Design review of the part shown in the three views and the two pictorial views. Dimensions are in mm from the part's minimum x, y and z. A direction names the side the tool comes from. Give positions to 0.01 mm unless a question says otherwise; leave off trailing zeros. Order: outer loops, then holes, each group sorted by start corner. A loop starts at its lowest first (then second) coordinate and runs counter-clockwise, first axis right, second up.
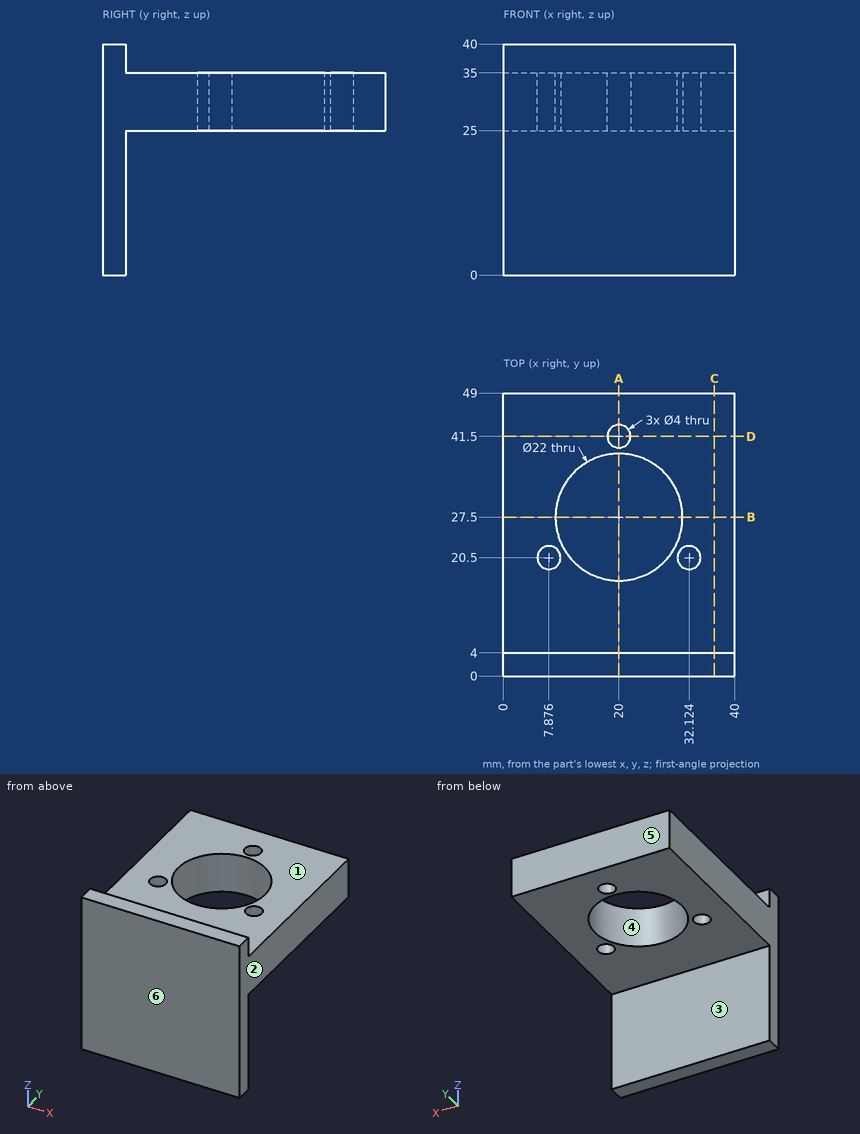
Item 1: For line 1 (Y direction, x = 20, z = 31.5); line 2 (X direction, y = 20, z = 29) (1 decimal); line 3 (X direction, y = 27, z = 30), list the stretches that pass through material, from the lowest coordinate up.
Values found:
line 1: y = 0 to 16.5, 38.5 to 39.5, 43.5 to 49
line 2: x = 0 to 5.9, 9.8 to 12, 28 to 30.2, 34.1 to 40
line 3: x = 0 to 9.01, 30.99 to 40
Item 2: Take a section at A-A (x = 20). Give the boundary of the cut face in (y, z), and give its area (3 significant figures).
Values found:
outline: (0, 0) - (4, 0) - (4, 25) - (16.5, 25) - (16.5, 35) - (4, 35) - (4, 40) - (0, 40) - close; (38.5, 25) - (39.5, 25) - (39.5, 35) - (38.5, 35) - close; (43.5, 25) - (49, 25) - (49, 35) - (43.5, 35) - close
area: 350 mm2
Item 3: For the marked faces 1, 2 and 3, list the 3-axis set-ups (+Z, -Z, +X, -X, +Y, -Y) from which the entire face can be reached by the end or side of a thin tool; tool diameter is ignored.
Values found:
face 1: +Z, +X, -X, +Y
face 2: +Z, -Z, +X, +Y, -Y
face 3: -Z, +X, -X, +Y
Item 4: Take a section at B-B (y = 27.5). Give the boundary of the cut face in (x, z), and give its area (3 significant figures).
Values found:
outline: (0, 25) - (9, 25) - (9, 35) - (0, 35) - close; (31, 25) - (40, 25) - (40, 35) - (31, 35) - close
area: 180 mm2
Item 5: Take a section at D-D (y = 41.5). Give the boundary of the cut face in (x, z).
Values found:
outline: (0, 25) - (18, 25) - (18, 35) - (0, 35) - close; (22, 25) - (40, 25) - (40, 35) - (22, 35) - close
Item 6: Take a section at C-C (x = 36.5). Give the boundary of the cut face in (y, z).
Values found:
outline: (0, 0) - (4, 0) - (4, 25) - (49, 25) - (49, 35) - (4, 35) - (4, 40) - (0, 40) - close
Item 7: Draft analysis for pull direction Y (two halves, no side actions). For the marked faces 4, 5 and 6, state which applies: released by +Y, released by -Y, zero draft, split by the parting line, or undercut.
Values found:
face 4: undercut
face 5: released by +Y
face 6: released by -Y
Item 8: Clearance check with flat-ended pins moving along their axes: pin 1 Ø20 at (x, z) = (29, 12.5) entering from +Y; pin 2 Ø12 at (x, y) = (31.5, 41.5) entering from -Z; pin 3 Ø2 at (x, y) = (22.5, 11.5) entering from +Z; pin 4 Ø3 at (x, y) = (20, 41.5) entering from -Z. State where each tip first meets the part, or that it passes through.
Values found:
pin 1: stops at y = 4
pin 2: stops at z = 25
pin 3: stops at z = 35
pin 4: passes through
